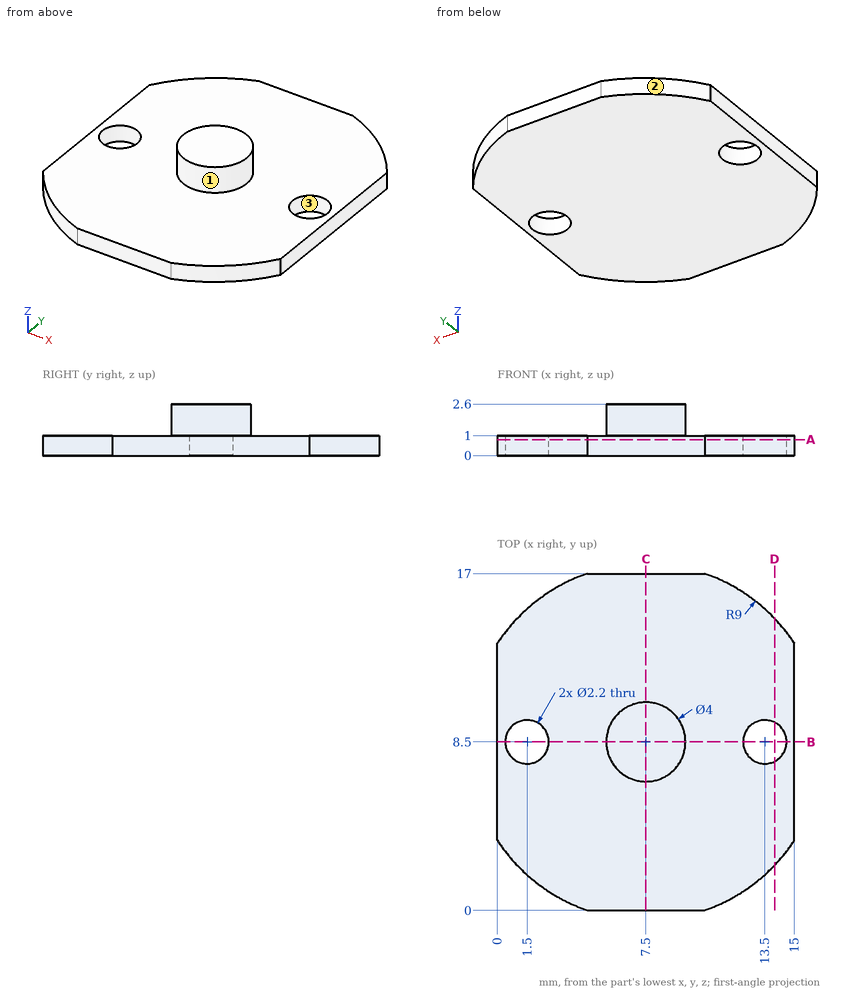
Could you check a few things on this drawing? It's one solid part, dimensions in mm from its lowest x, y, z. Give positions to 0.01 mm unless a question says otherwise; leave off trailing zeros. Order: outer loops, then holes, each group sorted by start corner. A loop starts at its lowest first (then second) coordinate and runs counter-clockwise, first axis right, second up. Notation, with made-up numbers: (69.5, -33.5) -> (86.5, -33.5) arc R17 cw to (86.5, -28.5) -> close; hole circle Ø10 at (81, 85). An arc over 180 degrees is marked (long way). Use CSV: the item, a comma, the result in double quotes. Start each with the question number.
Item 1: Suppose I cut it at A-A (z = 0.8). List the corners of the cut face in (x, y) for me, and give its area (3 significant figures).
Item 2: Suppose I cut it at D-D (x = 14). List the corners of the cut face in (y, z) for me, and give its area (3 significant figures).
Item 3: Suppose I cut it at B-B (y = 8.5). List the corners of the cut face in (x, z) for me, and give its area (3 significant figures).
Item 4: I'm going to push flat-ended pins straight in: P1, Ø1.3, axis at x = 1.5, y = 8.5, coming from the +Z side; P2, Ø1, axis at x = 2, z = 1, coming from the -Y side; P3, Ø4, axis at x = 9.5, y = 12.5, coming from the +Z side. Where does each tip first touch, or does it pass through?
Item 5: Thinking about a two-plate mould opening in X: for the marked faces 1, 2 and 3, which applies, pulls with the +X half, pulls with the -X half, needs draft (parallel to the pull), parting line crosses it, or undercut?
Item 6: Suppose I cut it at C-C (x = 7.5). List the corners of the cut face in (y, z) for me.
Item 7: If I drill on probe 1 along Z at (x, y) = (6.5, 6.5); probe 2 along Y at (x, z) = (13.5, 0.7); probe 3 along X at (y, z) = (14.5, 0.45), over which ranges is the centre line in solid material (lowest first)? Write a range as [from, to].
Answer block:
1,outline,"(0, 3.53) arc R9 ccw to (4.54, 0) -> (10.46, 0) arc R9 ccw to (15, 3.53) -> (15, 13.47) arc R9 ccw to (10.46, 17) -> (4.54, 17) arc R9 ccw to (0, 13.47) -> close; hole circle Ø2.2 at (1.5, 8.5); hole circle Ø2.2 at (13.5, 8.5)"
1,area,"223 mm^2"
2,outline,"(2.28, 0) -> (7.52, 0) -> (7.52, 1) -> (2.28, 1) -> close; (9.48, 0) -> (14.72, 0) -> (14.72, 1) -> (9.48, 1) -> close"
2,area,"10.5 mm^2"
3,outline,"(0, 0) -> (0.4, 0) -> (0.4, 1) -> (0, 1) -> close; (2.6, 0) -> (12.4, 0) -> (12.4, 1) -> (9.5, 1) -> (9.5, 2.6) -> (5.5, 2.6) -> (5.5, 1) -> (2.6, 1) -> close; (14.6, 0) -> (15, 0) -> (15, 1) -> (14.6, 1) -> close"
3,area,"17.0 mm^2"
4,P1,"passes through"
4,P2,"stops at y = 1.02"
4,P3,"stops at z = 1"
5,face 1,"parting line crosses it"
5,face 2,"pulls with the -X half"
5,face 3,"undercut"
6,outline,"(0, 0) -> (17, 0) -> (17, 1) -> (10.5, 1) -> (10.5, 2.6) -> (6.5, 2.6) -> (6.5, 1) -> (0, 1) -> close"
7,probe 1,"z = [0, 1]"
7,probe 2,"y = [1.79, 7.4], [9.6, 15.21]"
7,probe 3,"x = [0.79, 14.21]"
